Design review of the part built by this model. Coordinates are the model's own, in mm. A direction names the side the tool comes from. Coordinates: 2 decimals unless noted, no trailing zeros. Order: outer loops, then holes, each group sorted by start corner. A loop starts at its lowest first (then second) coordinate and runs counter-clockwise, first axis right, second up. Notation, with made-up numbers: (63, 2.25) -> (78, 2.25) arc R15 cw to (78, 11.25) -> close; hole circle Ø1 at (-6, 0). An arc over 180 degrees is marked (long way). Use a Markdown table: item, result. Add a question column.
Q1. Add section D-D (x = -3.5). State the section outline as (y, z) points, then the cut area to 3 significant figures.
Q2. Add section B-B (z = 0). State the section outline as (x, y) points.
Q3. Insertion check: pin 1 (1 mm diameter, centred on y = 2.5, z = -2.5, fed in from -X). The pin has a flat end and moves straight along its axis. Give the tip position at first contact, or say it passes through.
Q4. The part is to be moulded in two halves that separate along X. For faces 1 (the face through (3.65, 0.3, 2.8)), 2 (the face through (1.7, 0.6, 3.8)), 3 (the face through (0, 2, 2)), say which applies: pulls with the +X half, pulls with the -X half, needs draft (parallel to the pull), parting line crosses it, or undercut.
Q5. Add section A-A (x = 0). State the section outline as (y, z) points.
Q6. Add section C-C (y = 0.45). State the section outline as (x, z) points.
Q7. Machinability: for faces 4 (the face through (-2, 3, 1)), 5 (the face through (-0.867, 1.783, -3.905)), which of the approach directions +Z, -Z, +X, -X, +Y, -Y give a long, thin tool a straight path to every point of the face, cutting with its end or side? Answer none if there is none.
Q8. Wall thickness on probe 1 along Z at (x, y) = (0, 1.3); probe 2 along X at (y, z) = (0.2, -1.75): over which ranges is each line inside the solid? List them lowest first.
Autodesk Inventor part; units mm, degrees
ref_plane "YZ Plane" through (0, 0, 0) normal (1, 0, 0) x (0, 1, 0)
ref_plane "XZ Plane" through (0, 0, 0) normal (0, 1, 0) x (-1, 0, 0)
ref_plane "XY Plane" through (0, 0, 0) normal (0, 0, 1) x (1, 0, 0)
sketch "Sketch1" plane through (0, 0, 0) normal (0, 1, 0) x (-1, 0, 0)
  circle A0 centre (0, 0) radius 4.6
  dimension "d0" = 9.2
extrude "Extrusion1" add sketch "Sketch1" along normal blind 0.6
sketch "Sketch2" plane through (0, 0.6, 0) normal (0, 1, 0) x (1, 0, 0)
  circle A0 centre (0, 0) radius 4
  dimension "d3" = 8
extrude "Extrusion2" add sketch "Sketch2" along normal blind 2.4
sketch "Sketch3" plane through (0, 3, 0) normal (0, 1, 0) x (1, 0, 0)
  circle A0 centre (0, 0) radius 2
  dimension "d6" = 4
extrude "Extrusion3" cut sketch "Sketch3" against normal through all
equation "\"d7\" = d6"
properties part number "bearing_8_4_3_flanged"
Established:
| question | item | result |
|---|---|---|
| 1 | outline | (0, -2.98) -> (0.6, -2.98) -> (0.6, -1.94) -> (3, -1.94) -> (3, 1.94) -> (0.6, 1.94) -> (0.6, 2.98) -> (0, 2.98) -> close |
| 1 | area | 12.9 mm^2 |
| 2 | outline | (-4.6, 0) -> (-2, 0) -> (-2, 3) -> (-4, 3) -> (-4, 0.6) -> (-4.6, 0.6) -> close; (2, 0) -> (4.6, 0) -> (4.6, 0.6) -> (4, 0.6) -> (4, 3) -> (2, 3) -> close |
| 3 | pin 1 | x = -3.46 |
| 4 | face 1 | parting line crosses it |
| 4 | face 2 | needs draft |
| 4 | face 3 | undercut |
| 5 | outline | (0, -4.6) -> (0.6, -4.6) -> (0.6, -4) -> (3, -4) -> (3, -2) -> (0, -2) -> close; (0, 2) -> (3, 2) -> (3, 4) -> (0.6, 4) -> (0.6, 4.6) -> (0, 4.6) -> close |
| 6 | outline | circle Ø9.2 at (0, 0); hole circle Ø4 at (0, 0) |
| 7 | face 4 | +Z, -Z, +X, -X, +Y |
| 7 | face 5 | +Y |
| 8 | probe 1 | -4 to -2, 2 to 4 |
| 8 | probe 2 | -4.25 to -0.97, 0.97 to 4.25 |
